from build123d import *

# Parameters (mm, degrees)
SKETCH1_R           = 34.5
BOSS_EXTRUDE1_DEPTH = 30
SKETCH5_R           = 33.5
CUT_EXTRUDE2_DEPTH  = 18
CUT_REVOLVE3_ANGLE  = 180
CHAMFER1_SIZE       = 10


with BuildPart() as part:
    # Sketch1 → Boss-Extrude1 (new body)
    with BuildSketch(Plane.XY):
        Circle(SKETCH1_R)
    extrude(amount=BOSS_EXTRUDE1_DEPTH)

    # Sketch5 → Cut-Extrude2 (cut)
    with BuildSketch(Plane.XY.offset(30)):
        Circle(SKETCH5_R)
    extrude(amount=-CUT_EXTRUDE2_DEPTH, mode=Mode.SUBTRACT)

    # Sketch7 → Cut-Revolve3 (revolve, cut)
    with BuildSketch(Plane.XY.offset(12)):
        with BuildLine():
            Line((-16.25, 0), (16.25, 0))
            ThreePointArc((16.25, 0), (0, 16.25), (-16.25, 0))
        make_face()
    revolve(axis=Axis((-16.25, 0, 12), (-1, 0, 0)), revolution_arc=CUT_REVOLVE3_ANGLE, mode=Mode.SUBTRACT)

    # Chamfer1
    chamfer1_edges = [part.edges().sort_by_distance(p)[0] for p in [
        (-34.5, 0, 0),
    ]]
    chamfer(chamfer1_edges, length=CHAMFER1_SIZE)


solid = part.part
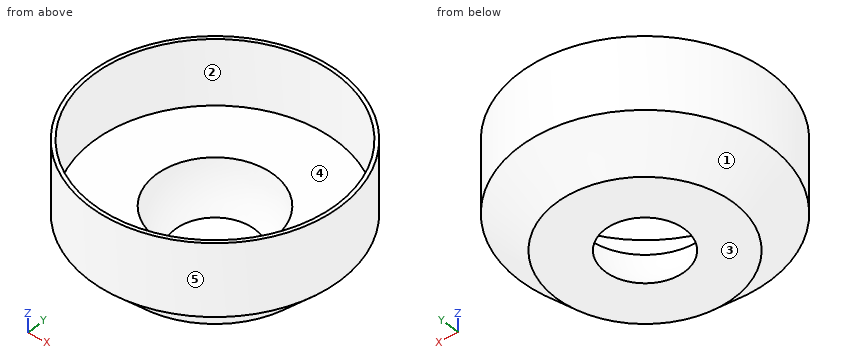
Can you work these out from the model? Positions are in its coordinate system, mm. Face numbers are marked on the shaded views. A direction names the side the tool comes from. Coordinates: 2 decimals unless noted, no trailing zeros. Order: outer loops, then holes, each group sorted by start corner. A loop starts at its lowest first (then second) coordinate and runs counter-clockwise, first axis right, second up. Notation, with made-up numbers: (9, 32) - (64, 32) arc R10 ccw to (64, 47) - close; hole circle Ø4 at (47, 72). An arc over 180 degrees is marked (long way). Answer as a JSON object with one key per item and string values. Group by question number.
Q1. Imagine slicing it at D-D (z = 5.75). Please give me the cut outline in (x, y).
Q2. Imagine slicing it at A-A (x = 0). Please give me the cut outline in (y, z).
Q3. On a 3-axis mill with a long thin cutter (end or side, diameter ignored), from which of +Z, -Z, +X, -X, +Y, -Y can I reach the whole of each face in a straight line? I mean the marked faces 1 and 2. Say none if no direction works.
Q4. Will these pins go through, and if not, where does the flat tip stop? P1, Ø2, axis at y = -24.5, z = 7.5, coming from the +X side; P2, Ø2, axis at x = 15, z = 20, coming from the +Y side; P3, Ø6, axis at x = -21, z = 10, coming from the +Y side.
Q5. I need wall thicknesses on line 1 (Y direction, x = 0, z = 19.25); line 2 (Z direction, x = -17.5, y = 14.5); line 3 (Y direction, x = -28, z = 19.5). Which ranges of each line are inside material? Lowest first, please. Write a range as from..to.
Q6. Imagine slicing it at C-C (z = 13). Please give me the cut outline in (x, y), and give its area (3 significant figures).
Q7. We'd pull the mould along Y, two halves only. Please class the marked faces 3, 4 and 5: +Y half, -Y half, draft (parallel to the pull), parting line (faces both ways), or undercut.
Determined:
{
 "1": {"outline": "circle Ø60.5 at (0, 0); hole circle Ø30 at (0, 0)"},
 "2": {"outline": "(-34.5, 10) - (-24.5, 0) - (-10.96, 0) arc R16.25 cw to (-16.25, 12) - (-33.5, 12) - (-33.5, 30) - (-34.5, 30) - close; (10.96, 0) - (24.5, 0) - (34.5, 10) - (34.5, 30) - (33.5, 30) - (33.5, 12) - (16.25, 12) arc R16.25 cw to start"},
 "3": {"face 1": "-Z", "face 2": "+Z"},
 "4": {"P1": "stops at x = 22.46", "P2": "stops at y = 31.53", "P3": "stops at y = 29.43"},
 "5": {"line 1": "y = -34.5..-33.5, 33.5..34.5", "line 2": "z = 0..12", "line 3": "y = -20.16..-18.39, 18.39..20.16"},
 "6": {"outline": "circle Ø69 at (0, 0); hole circle Ø67 at (0, 0)", "area": "214 mm2"},
 "7": {"face 3": "draft", "face 4": "undercut", "face 5": "parting line"}
}
